Can you work these out from the drawing? Everything is in mm from the part's minimum corner. A direction names the side the tool comes from. Round coordinates to 2 decimals unless told otherwise and drop trailing zeros. Order: outer loops, then holes, each group sorted by start corner. A loop starts at its lowest first (then second) coordinate and runs counter-clockwise, first axis right, second up. Notation, with made-up numbers: (67.5, 41.5) - (101.5, 41.5) arc R22 cw to (101.5, 48.5) - close; hole circle Ø6 at (73, -21). An arc over 180 degrees is marked (long way). Write item = value, one per line.
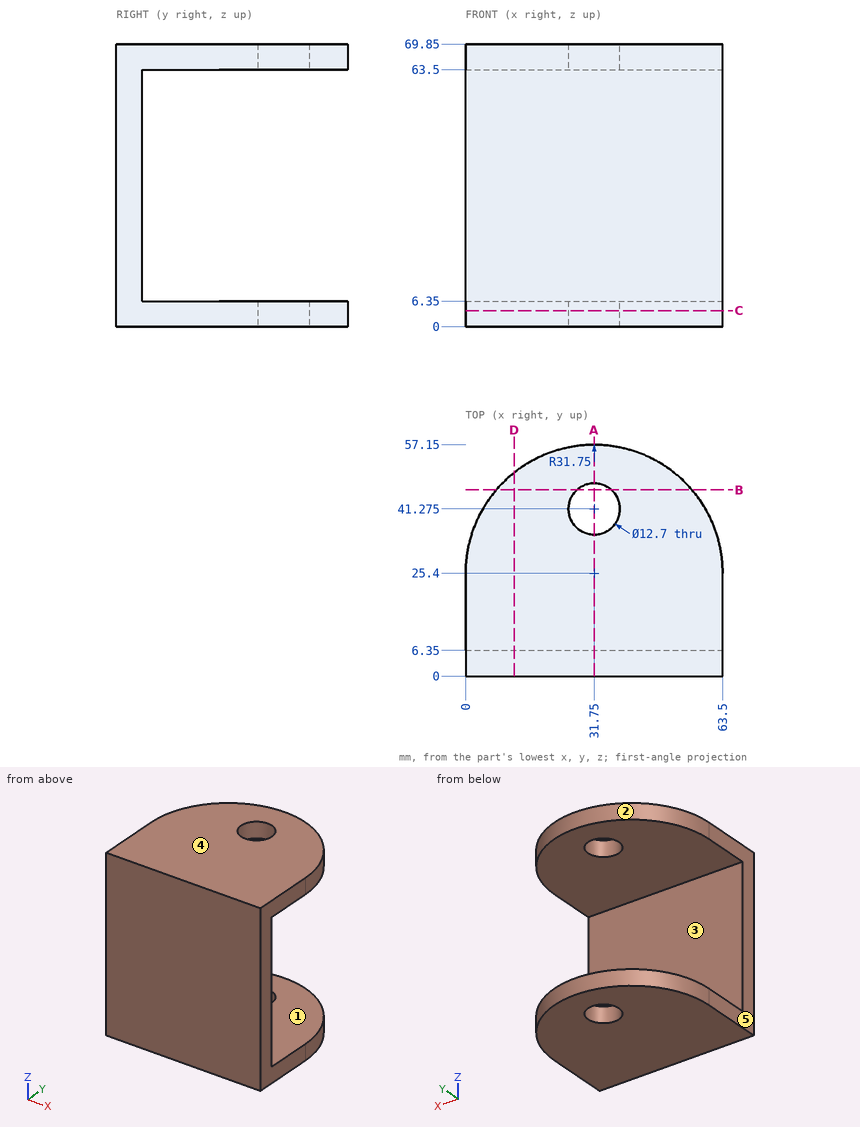
(1) If we section it at C-C (z = 4): Write out the boundary of the cut face in (x, y) (3 decimals).
Computed:
outline = (0, 0) - (63.5, 0) - (63.5, 25.4) arc R31.75 ccw to (0, 25.4) - close; hole circle Ø12.7 at (31.75, 41.275)
(2) If we section it at B-B (y = 46): Write out the boundary of the cut face in (x, z), plus the area to 3 significant figures.
Computed:
outline = (7.59, 0) - (27.51, 0) - (27.51, 6.35) - (7.59, 6.35) - close; (7.59, 63.5) - (27.51, 63.5) - (27.51, 69.85) - (7.59, 69.85) - close; (35.99, 0) - (55.91, 0) - (55.91, 6.35) - (35.99, 6.35) - close; (35.99, 63.5) - (55.91, 63.5) - (55.91, 69.85) - (35.99, 69.85) - close
area = 506 mm^2
(3) If we section it at A-A (x = 31.75): Write out the boundary of the cut face in (y, z) (3 decimals), plus the area to 3 significant figures.
Computed:
outline = (0, 0) - (34.925, 0) - (34.925, 6.35) - (6.35, 6.35) - (6.35, 63.5) - (34.925, 63.5) - (34.925, 69.85) - (0, 69.85) - close; (47.625, 0) - (57.15, 0) - (57.15, 6.35) - (47.625, 6.35) - close; (47.625, 63.5) - (57.15, 63.5) - (57.15, 69.85) - (47.625, 69.85) - close
area = 927 mm^2
(4) On a 3-axis mill with a long thin cutter (end or side, diameter ignored), from which of +Z, -Z, +X, -X, +Y, -Y can I reach the whole of each face in a straight line? I mean the marked faces 1 and 2. Say none if no direction works.
Computed:
face_1 = +X, -X, +Y
face_2 = +Z, -Z, +Y
(5) Will these pins go through, and if not, where does the flat tip stop? P1, Ø16.5, axis at x = 31.75, y = 41.275, coming from the -Z side; P2, Ø8, axis at x = 55.5, z = 9.5, coming from the +Y side; P3, Ø2, axis at x = 19, z = 21, coming from the +Y side.
Computed:
P1 = 0
P2 = 48.96
P3 = 6.35
(6) If we section it at D-D (x = 12): Write out the boundary of the cut face in (y, z).
Computed:
outline = (0, 0) - (50.26, 0) - (50.26, 6.35) - (6.35, 6.35) - (6.35, 63.5) - (50.26, 63.5) - (50.26, 69.85) - (0, 69.85) - close
(7) Thinking about a two-plate mould opening in Z: for the marked faces 3, 4 and 5, which applies, +Z half, -Z half, draft (parallel to the pull), parting line (faces both ways), or undercut?
Computed:
face_3 = undercut
face_4 = +Z half
face_5 = draft
(8) If I drill on line 1 (Y direction, x = 31.75, z = 65.5) (3 decimals); line 2 (Z direction, x = 24.5, y = 40); line 3 (Y direction, x = 40, z = 51), over which ranges is the centre line in solid material (lowest first)? Write a range as from..to.
Computed:
line_1 = 0..34.925, 47.625..57.15
line_2 = 0..6.35, 63.5..69.85
line_3 = 0..6.35
